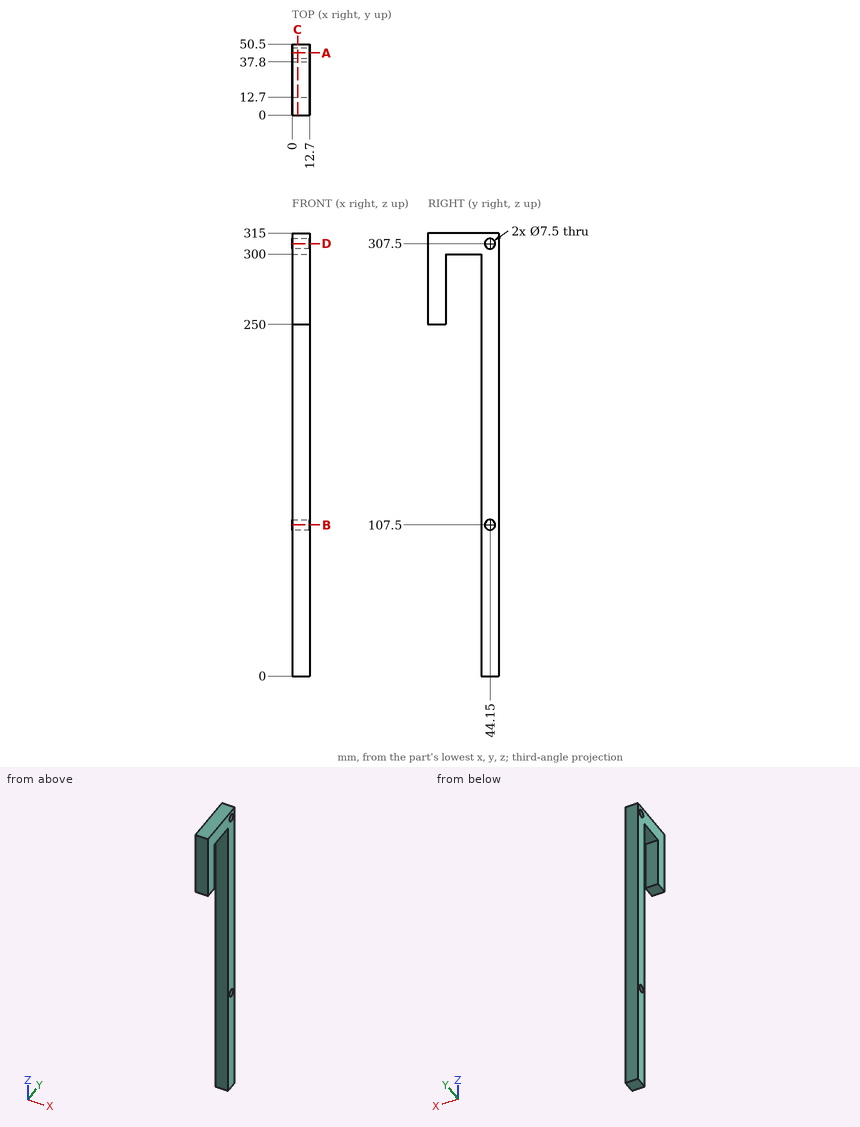
Drawing for the job (mm, zero at the part's lowest x, y, z). Give positions to 0.01 mm unless a question says otherwise; leave off trailing zeros. Write each loop counter-clockwise with the first axis right and the second up, starting at its lowest first coordinate (ties: lowest second). Pieces come first, ordered by that corner, then holes. Notation, with made-up numbers: M 67.5,8 L 122.5,8 A20 ccw 122.5,28 Z; hole C -1,8 d11. An arc over 180 degrees is marked long. Return JSON: item names as keys, results as strings. Group by question number.
(1) Band-saw the part on A-A (y = 44.15). Give the cut face in (x, z).
(2) Flat gauge pins, fed straight in: pin 1 Ø4 at (x, z) = (7, 107.5) entering from -Y; pin 2 Ø6.5 at (x, y) = (6, 4.5) entering from -Z; pin 3 Ø4 at (x, y) = (8.5, 29) entering from -Z. Where does each tip first touch, or does it go through?
(3) Drill centre lines: L1, parallel to Y at x = 5, z = 107.5; L2, parallel to Y at x = 3.75, z = 286; L3, parallel to Y at x = 3, z = 138.5. Where is each one in solid material? Low to high. Write a range as [from, to].
(4) Band-saw the part on B-B (z = 107.5). Give the cut face in (x, y).
(5) Band-saw the part on D-D (z = 307.5). Give the cut face in (x, y).
(6) Band-saw the part on C-C (x = 4). Give the cut face in (y, z).
Entries:
{
 "1": {"outline": "M 0,0 L 12.7,0 L 12.7,103.75 L 0,103.75 Z; M 0,111.25 L 12.7,111.25 L 12.7,303.75 L 0,303.75 Z; M 0,311.25 L 12.7,311.25 L 12.7,315 L 0,315 Z"},
 "2": {"pin 1": "stops at y = 37.8", "pin 2": "stops at z = 250", "pin 3": "stops at z = 300"},
 "3": {"L1": "y = [37.8, 40.4], [47.9, 50.5]", "L2": "y = [0, 12.7], [37.8, 50.5]", "L3": "y = [37.8, 50.5]"},
 "4": {"outline": "M 0,37.8 L 12.7,37.8 L 12.7,40.4 L 0,40.4 Z; M 0,47.9 L 12.7,47.9 L 12.7,50.5 L 0,50.5 Z"},
 "5": {"outline": "M 0,0 L 12.7,0 L 12.7,40.4 L 0,40.4 Z; M 0,47.9 L 12.7,47.9 L 12.7,50.5 L 0,50.5 Z"},
 "6": {"outline": "M 0,250 L 12.7,250 L 12.7,300 L 37.8,300 L 37.8,0 L 50.5,0 L 50.5,315 L 0,315 Z; hole C 44.15,107.5 d7.5; hole C 44.15,307.5 d7.5"}
}
